from build123d import *

# Parameters (mm, degrees)
F1_DEPTH  = 20
F3_DEPTH  = 25
F4_DEPTH  = 25
F6_DEPTH  = 25
F7_DEPTH  = 25
F2_R      = 5
F8_DEPTH  = 30
F5_W      = 5
F5_H      = 5
F9_DEPTH  = 50
F10_DEPTH = 50


with BuildPart() as f1:
    # F0 (on Front) → F1 (new body)
    with BuildSketch(Plane.XZ):
        Polygon((0, 20), (0, 0), (18.7821621219, 0), (18.7821621219, 5), (30, 5), (30, 20), align=None)
    extrude(amount=-F1_DEPTH)

    # F2 (on face) → F3 (cut)
    with BuildSketch(Plane.XY.offset(20)):
        with BuildLine():
            ThreePointArc((0, 10), (2.9289321881, 17.0710678119), (10, 20))
            Line((10, 20), (0, 20))
            Line((0, 20), (0, 10))
        make_face()
    extrude(amount=-F3_DEPTH, mode=Mode.SUBTRACT)

    # F2 (on face) → F4 (cut)
    with BuildSketch(Plane.XY.offset(20)):
        with BuildLine():
            Line((0, 0), (10, 0))
            ThreePointArc((10, 0), (2.9289321881, 2.9289321881), (0, 10))
            Line((0, 10), (0, 0))
        make_face()
    extrude(amount=-F4_DEPTH, mode=Mode.SUBTRACT)

    # F2 (on face) → F6 (cut)
    with BuildSketch(Plane.XY.offset(20)):
        Polygon((30, 20), (25, 20), (30, 15), align=None)
    extrude(amount=-F6_DEPTH, mode=Mode.SUBTRACT)

    # F2 (on face) → F7 (cut)
    with BuildSketch(Plane.XY.offset(20)):
        Polygon((30, 5), (25, 0), (30, 0), align=None)
    extrude(amount=-F7_DEPTH, mode=Mode.SUBTRACT)

    # F2 (on face) → F8 (cut)
    with BuildSketch(Plane.XY.offset(20)):
        with Locations((10, 10)):
            Circle(F2_R)
    extrude(amount=-F8_DEPTH, mode=Mode.SUBTRACT)

    # F5 (on face) → F9 (cut)
    with BuildSketch(Plane.YZ.offset(30)):
        with Locations((10, 7.5)):
            Rectangle(F5_W, F5_H)
    extrude(amount=-F9_DEPTH, mode=Mode.SUBTRACT)

    # F5 (on face) → F10 (cut)
    with BuildSketch(Plane.YZ.offset(30)):
        with Locations((10, 2.5)):
            Rectangle(F5_W, F5_H)
    extrude(amount=-F10_DEPTH, mode=Mode.SUBTRACT)


solid = f1.part
Input: part model. Units: mm. Frame: model coordinates. A direction names the side the tool comes from. Round coordinates to 2 decimals unless told otherwise and drop trailing zeros. Loops run counter-clockwise (first coordinate to the right, second up) from the corner with the lowest first, then second, coordinate; pieces in that order, holes last. Notation, with made-up numbers: (40.5, 73) -> (91.5, 73) arc R19 cw to (91.5, 105) -> close; hole circle Ø1 at (42, -23). An arc over 180 degrees is marked (long way). Answer as a JSON object with one key per item and string values. Group by question number.
1) Section query A-A on z = 4. Output: boundary loops of the cut face in (x, y).
2) Pin query (flat end, axial travel): pin 1 (6 mm diameter, centred on x = 10, y = 10, fed in from -Z); pin 2 (2.5 mm diameter, centred on x = 25, y = 10, fed in from -Z); pin 3 (1.5 mm diameter, centred on y = 17.5, z = 1.5, fed in from +X); pin 4 (1 mm diameter, centred on y = 17.5, z = 13, fed in from +X). Return the tip coordinate at first contact, or that it passes through.
3) Section query C-C on z = 15.25. Output: boundary loops of the cut face in (x, y).
4) Reachability of faces 1 (the flat face through (3, 10, 10)), 2 (the flat face through (17, 20, 10)), 3 (the flat face through (23, 4, 5)) from +Z, -Z, +X, -X, +Y, -Y: full face, straight path, thin tool, end or side. Return the list, or none.
5) Section query D-D on y = 8.75. Output: boundary loops of the cut face in (x, z).
6) Section query B-B on x = 10.5. Output: boundary loops of the cut face in (y, z).
7) Ray query, L1, parallel to Y at x = 10, z = 13.5; L2, parallel to Y at x = 23.25, z = 6.5; L3, parallel to Z at x = 26.5, y = 5. Return the intervals inside material, ascending.
Reply:
{
 "1": {"outline": "(0.32, 7.5) arc R10 ccw to (10, 0) -> (18.78, 0) -> (18.78, 7.5) -> (14.33, 7.5) arc R5 cw to (5.67, 7.5) -> close; (0.32, 12.5) -> (5.67, 12.5) arc R5 cw to (14.33, 12.5) -> (18.78, 12.5) -> (18.78, 20) -> (10, 20) arc R10 ccw to start"},
 "2": {"pin 1": "passes through", "pin 2": "stops at z = 10", "pin 3": "stops at x = 18.78", "pin 4": "stops at x = 28"},
 "3": {"outline": "(10, 0) -> (25, 0) -> (30, 5) -> (30, 15) -> (25, 20) -> (10, 20) arc R10 ccw to start; hole circle Ø10 at (10, 10)"},
 "4": {"face 1": "-Z, +X, -X", "face 2": "+Z, -Z, +X, -X, +Y", "face 3": "-Z, +X, +Y, -Y"},
 "5": {"outline": "(0.08, 10) -> (5.16, 10) -> (5.16, 20) -> (0.08, 20) -> close; (14.84, 10) -> (30, 10) -> (30, 20) -> (14.84, 20) -> close"},
 "6": {"outline": "(0, 0) -> (5.03, 0) -> (5.03, 20) -> (0, 20) -> close; (14.97, 0) -> (20, 0) -> (20, 20) -> (14.97, 20) -> close"},
 "7": {"L1": "y = 0 to 5, 15 to 20", "L2": "y = 0 to 7.5, 12.5 to 20", "L3": "z = 5 to 20"}
}
